```python
from build123d import *

# Parameters (mm, degrees)
BOTTOM_BLADE_EXTRUDE_DEPTH        = 10
BOTTOM_BLADE_CUT_1_SIZE           = 1
BOTTOM_BLADE_CUT_2_SIZE           = 1
SKETCH3_R                         = 1
HOLE_FOR_SCREW_BOTTOM_BLADE_DEPTH = 20


with BuildPart() as part:
    # Sketch2 → Bottom Blade Extrude (new body)
    with BuildSketch(Plane(origin=(0, 0, 0), x_dir=(1, 0, 0), z_dir=(0, 1, 0))):
        Polygon((-27.237322503, 0), (12.762677497, 0), (17.762677497, -5), (32.762677497, -5), (32.762677497, -4), (18.17689106, -4), (13.17689106, 1), (-27.651536065, 1), (-32.651536065, -4), (-47.237322503, -4), (-47.237322503, -5), (-32.237322503, -5), align=None)
    extrude(amount=BOTTOM_BLADE_EXTRUDE_DEPTH)

    # Bottom Blade Cut 1
    bottom_blade_cut_1_edges = [part.edges().sort_by_distance(p)[0] for p in [
        (-30.151536065, 10, 1.5),
        (-39.944429284, 10, 4),
    ]]
    chamfer(bottom_blade_cut_1_edges, length=BOTTOM_BLADE_CUT_1_SIZE - 0.0001)  # a hair under: the kernel refuses the full size

    # Bottom Blade Cut 2
    bottom_blade_cut_2_edges = [part.edges().sort_by_distance(p)[0] for p in [
        (15.67689106, 0, 1.5),
        (25.469784279, 0, 4),
    ]]
    chamfer(bottom_blade_cut_2_edges, length=BOTTOM_BLADE_CUT_2_SIZE - 0.0001)  # a hair under: the kernel refuses the full size

    # Sketch3 → Hole for Screw ( Bottom Blade) (cut)
    with BuildSketch(Plane.XY):
        with Locations((-7.237322503, 5)):
            Circle(SKETCH3_R)
    extrude(amount=-HOLE_FOR_SCREW_BOTTOM_BLADE_DEPTH, mode=Mode.SUBTRACT)


solid = part.part
```
Model file for the job. Use its own axes, mm. A direction names the side the tool comes from. Coordinates: 2 decimals unless noted, no trailing zeros. Order: outer loops, then holes, each group sorted by start corner. A loop starts at its lowest first (then second) coordinate and runs counter-clockwise, first axis right, second up. Notation, with made-up numbers: (-6.5, -9) -> (11.5, -9) arc R29 ccw to (11.5, 16) -> close; hole circle Ø3 at (4.25, -37). An arc over 180 degrees is marked (long way). Answer as a JSON object with one key per item and string values. Group by question number.
1) Cut at A-A, the plane y = 5. Write the cut outline in (x, z), then the cut area to 3 significant figures.
2) Drill centre lines: L1, parallel to Z at x = -13.5, y = 6.5; L2, parallel to Z at x = 27.5, y = 8.75; L3, parallel to X at y = 5.25, z = 0.5. Where is each one in solid material? Low to high.
3) Flat gauge pins, fed straight in: pin 1 (3 mm diameter, centred on x = 12, y = 7, fed in from +Z); pin 2 (5 mm diameter, centred on x = -16, y = 7.5, fed in from +Z). Where does each tip first touch, or does it go through?
4) Which spindle directions (+Z, -Z, +X, -X, +Y, -Y) get a long thin tool onto all of the face, cutting with end or side? Do faces 4 (the face through (26, 5, 4)), 5 (the face through (-40, 4, 4)), 6 (the face through (15.23, 4.93, 2.47)). Say none if no direction does.
5) Pull direction Y, two halves, no side cores. Call faces 1 (the face through (-6.284, 5.3, -0.493)), 2 (the face through (1.5, 10, -0.2)), 3 (the face through (-8, 6, 0)): +Y half, -Y half, draft (parallel to the pull), parting line (faces both ways), or undercut.
Check values:
{
 "1": {"outline": "(-47.24, 4) -> (-32.65, 4) -> (-27.65, -1) -> (-8.24, -1) -> (-8.24, 0) -> (-27.24, 0) -> (-32.24, 5) -> (-47.24, 5) -> close; (-6.24, -1) -> (13.18, -1) -> (18.18, 4) -> (32.76, 4) -> (32.76, 5) -> (17.76, 5) -> (12.76, 0) -> (-6.24, 0) -> close", "area": "82.1 mm²"},
 "2": {"L1": "z = -1 to 0", "L2": "z = 4 to 5", "L3": "x = -29.15 to -27.74, 13.26 to 14.68"},
 "3": {"pin 1": "stops at z = 0.74", "pin 2": "stops at z = 0"},
 "4": {"face 4": "-Z, +X, +Y, -Y", "face 5": "-Z, -X, +Y, -Y", "face 6": "+Z, +Y, -Y"},
 "5": {"face 1": "undercut", "face 2": "+Y half", "face 3": "draft"}
}
